Input: dimensioned drawing with shaded views. Units: mm. Origin: part minimum x, y, z. A direction names the side the tool comes from. Give positions to 0.01 mm unless a question says otherwise; leave off trailing zeros. Write each loop counter-clockwise with the first axis right and the second up, starting at its lowest first coordinate (ties: lowest second). Pieces come first, ordered by that corner, then holes. Notation, with made-up numbers: (-37, -16) -> (0, -16) arc R20 ccw to (0, -11) -> close; hole circle Ø11 at (13.25, -0.75). An arc over 180 degrees is marked (long way). Return JSON: item names as keys, results as strings. Group by question number.
Item 1: Line query: line 1 (Y direction, x = 15, z = 11); line 2 (X direction, y = 15.5, z = 3); line 3 (Z direction, x = 13, y = 8). Output: solid intervals per line, ascending. Write a range as [from, to].
Item 2: Pin query (flat end, axial travel): P1, Ø2, axis at x = 25, z = 3, coming from the -Y side; P2, Ø1, axis at y = 25.5, z = 9.5, coming from the +X side; P3, Ø1, axis at y = 14, z = 2.5, coming from the -X side. Return the tip coordinate at first contact, or that it passes through.
Item 3: Section D-D, the plane z = 5.5. Return loops of the section in (x, y), then the cut area to 3 significant figures.
Item 4: Section B-B, the plane z = 2. Return loops of the section in (x, y).
Item 5: Section C-C, the plane y = 15. Return loops of the section in (x, z), then the cut area to 3 significant figures.
Item 6: Section A-A, the plane x = 15. Return loops of the section in (y, z).
Item 7: Mould query, pull axis Y, two halves, no side actions, for the marked faces 4, 5 and 6. Classes: released by +Y, released by -Y, zero draft, split by the parting line, or undercut.
Item 8: Set-up query: the marked faces 1, 2 and 3. Return all of +Z, -Z, +X, -X, +Y, -Y with unobstructed straight access to the full face (end or side cutting, diameter ignored); none if empty.
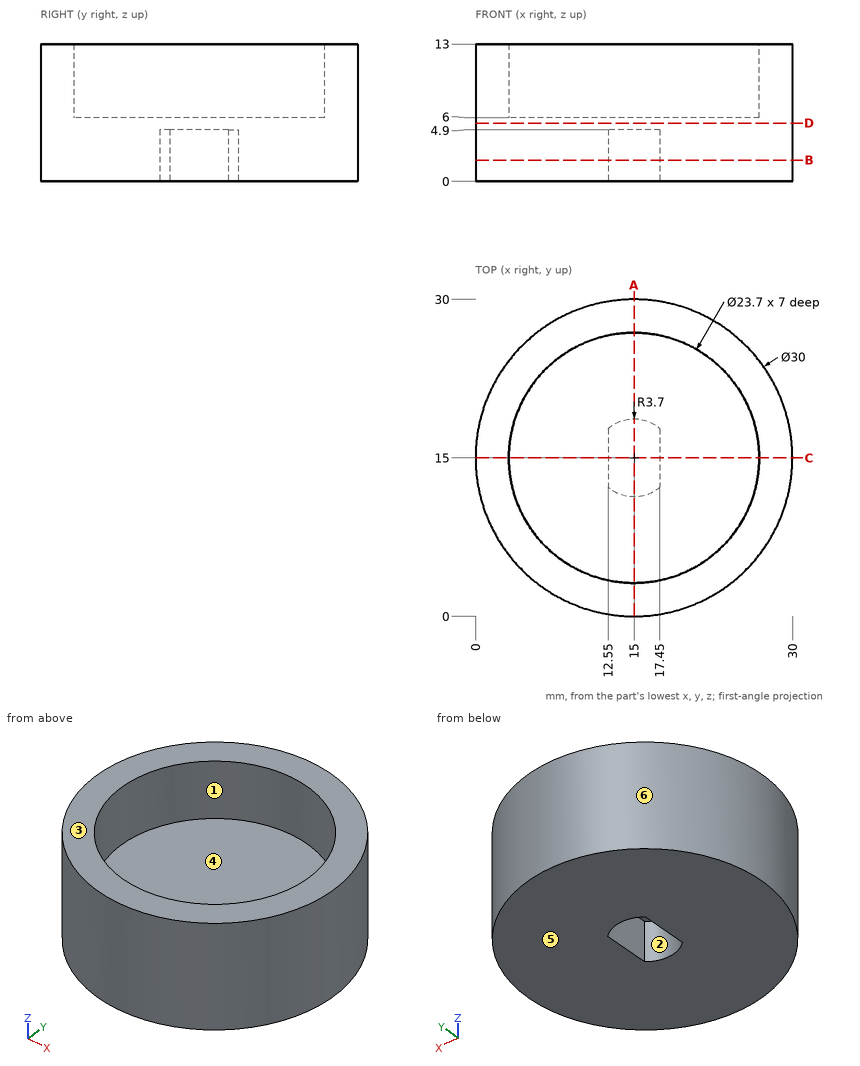
Answer below:
{
 "1": {"line 1": "y = [0, 3.15], [26.85, 30]", "line 2": "x = [0.01, 12.55], [17.45, 29.99]", "line 3": "z = [0, 6]"},
 "2": {"P1": "stops at y = 3", "P2": "stops at x = 26.18", "P3": "stops at x = 0.01"},
 "3": {"outline": "circle Ø30 at (15, 15)", "area": "707 mm2"},
 "4": {"outline": "circle Ø30 at (15, 15); hole (12.55, 12.23) arc R3.7 ccw to (17.45, 12.23) -> (17.45, 17.77) arc R3.7 ccw to (12.55, 17.77) -> close"},
 "5": {"outline": "(0, 0) -> (12.55, 0) -> (12.55, 4.9) -> (17.45, 4.9) -> (17.45, 0) -> (30, 0) -> (30, 13) -> (26.85, 13) -> (26.85, 6) -> (3.15, 6) -> (3.15, 13) -> (0, 13) -> close", "area": "200 mm2"},
 "6": {"outline": "(0, 0) -> (11.3, 0) -> (11.3, 4.9) -> (18.7, 4.9) -> (18.7, 0) -> (30, 0) -> (30, 13) -> (26.85, 13) -> (26.85, 6) -> (3.15, 6) -> (3.15, 13) -> (0, 13) -> close"},
 "7": {"face 4": "undercut", "face 5": "zero draft", "face 6": "split by the parting line"},
 "8": {"face 1": "+Z", "face 2": "-Z", "face 3": "+Z, +X, -X, +Y, -Y"}
}
